Input: part model. Units: mm. Frame: model coordinates. Face numbers are marked on the shaded views. A direction names the side the tool comes from. Give positions to 0.01 mm unless a question says otherwise; leave off trailing zeros. Loops run counter-clockwise (first coordinate to the right, second up) from the corner with the lowest first, then second, coordinate; pieces in that order, holes last. Notation, with made-up numbers: M 46.25,59 L 51.25,59 A6 cw 51.25,67 Z; hole C 69.5,37.5 d2. An arc over 180 degrees is marked long. Answer as a JSON object with one key per item and string values. Group by question number.
1) Ray query, L1, parallel to X at y = 9, z = -96; L2, parallel to Z at x = -37.2, y = 10; L3, parallel to X at y = 14.25, z = -99. Return the intervals inside material, ascending.
2) First-contact query: P1, Ø6.5, axis at y = 10, z = -100, coming from the -X side; P2, Ø4, axis at x = 23, y = 8.5, coming from the -Z side; P3, Ø3, axis at y = 12, z = -98, coming from the +X side. Flat tips, straight axial feed; report the tip coordinate or a pass-through.
3) Access query for the marked faces 1 and 2. Directions: +Z, -Z, +X, -X, +Y, -Y. A direction counts if a zero-diameter tool reaches every point of the face in a straight line with its end or side. Return the directions, or none.
4) Section query B-B on x = 28.5. Return loops of the section in (y, z).
5) Section query A-A on z = -89. Return loops of the section in (x, y), plus the area to 3 significant figures.
6) Section query D-D on x = -7.5. Return loops of the section in (y, z), plus the area to 3 significant figures.
7) Section query C-C on z = -32. Return loops of the section in (x, y), plus the area to 3 significant figures.
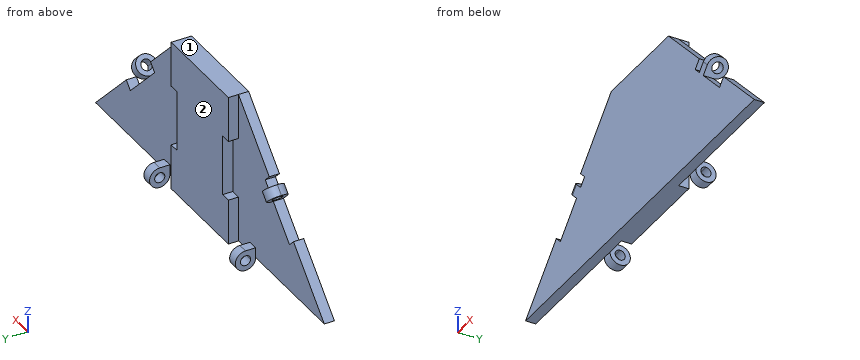
from build123d import *

# Parameters (mm, degrees)
BOSS_EXTRUDE1_DEPTH = 10
SKETCH2_W           = 5
SKETCH2_H           = 30
CUT_EXTRUDE1_DEPTH  = 5
CUT_EXTRUDE2_REACH  = 143.774
BOSS_EXTRUDE2_START = 5
BOSS_EXTRUDE2_DEPTH = 5
BOSS_EXTRUDE3_START = 10
BOSS_EXTRUDE3_DEPTH = 5


with BuildPart() as part:
    # Sketch1 → Boss-Extrude1 (new body)
    with BuildSketch(Plane(origin=(0, 0, 0), x_dir=(1, 0, 0), z_dir=(0, 1, 0))):
        Polygon((-25, 25), (-100, 100), (100, 100), (25, 25), align=None)
    extrude(amount=BOSS_EXTRUDE1_DEPTH)

    # Sketch2 → Cut-Extrude1 (cut)
    with BuildSketch(Plane(origin=(0, 10, 0), x_dir=(1, 0, 0), z_dir=(0, 1, 0))):
        Polygon((-25, 25), (-25, 47.5), (-25, 77.5), (-25, 100), (-100, 100), (-73.106601718, 73.106601718), (-69.571067812, 76.642135624), (-48.357864376, 55.428932188), (-51.893398282, 51.893398282), align=None)
        with Locations((-22.5, 62.5)):
            Rectangle(SKETCH2_W, SKETCH2_H)
    cut_extrude1 = extrude(amount=-CUT_EXTRUDE1_DEPTH, mode=Mode.SUBTRACT)

    # Sketch2_4 → Cut-Extrude2 (cut, up to next)
    with BuildSketch(Plane(origin=(0, 10, 0), x_dir=(1, 0, 0), z_dir=(0, 1, 0)), mode=Mode.PRIVATE) as cut_extrude2_sk1:
        Polygon((-73.106601718, 73.106601718), (-51.893398282, 51.893398282), (-48.357864376, 55.428932188), (-69.571067812, 76.642135624), align=None)
    cut_extrude2_tool1 = extrude(cut_extrude2_sk1.sketch, amount=-CUT_EXTRUDE2_REACH, mode=Mode.PRIVATE) & part.part
    cut_extrude2 = cut_extrude2_tool1.solids().sort_by_distance((-60.732233, 10, -64.267767))[0]
    add(cut_extrude2, mode=Mode.SUBTRACT)

    # Sketch3 → Boss-Extrude2 (add)
    with BuildSketch(Plane(origin=(-51.893398282, 0, -51.893398282), x_dir=(-0.7071067811865461, 0, 0.7071067811865489), z_dir=(-0.7071067811865489, 0, -0.7071067811865461)).offset(BOSS_EXTRUDE2_START)):
        with BuildLine():
            ThreePointArc((0, 0), (-3.535533906, 1.464466094), (-5, 5))
            Line((-5, 5), (-5, 0))
            Line((-5, 0), (0, 0))
        make_face()
        with BuildLine():
            ThreePointArc((0, 0), (3.535533906, 1.464466094), (5, 5))
            ThreePointArc((5, 5), (0, 10), (-5, 5))
            Line((-5, 5), (-2.634477445, 5))
            ThreePointArc((-2.634477445, 5), (0, 7.634477445), (2.634477445, 5))
            ThreePointArc((2.634477445, 5), (1.862856866, 3.137143134), (0, 2.365522555))
            Line((0, 2.365522555), (0, 0))
        make_face()
        with BuildLine():
            Line((-2.634477445, 5), (-5, 5))
            ThreePointArc((-5, 5), (-3.535533906, 1.464466094), (0, 0))
            Line((0, 0), (0, 2.365522555))
            ThreePointArc((0, 2.365522555), (-1.862856866, 3.137143134), (-2.634477445, 5))
        make_face()
    boss_extrude2 = extrude(amount=BOSS_EXTRUDE2_DEPTH)

    # Sketch4 → Boss-Extrude3 (add)
    with BuildSketch(Plane.ZY.offset(25).offset(BOSS_EXTRUDE3_START)):
        with BuildLine():
            Line((-97.5, 10), (-95, 10))
            ThreePointArc((-95, 10), (-103.535533906, 13.535533906), (-100, 5))
            Line((-100, 5), (-100, 7.5))
            ThreePointArc((-100, 7.5), (-101.767766953, 11.767766953), (-97.5, 10))
        make_face()
        with BuildLine():
            ThreePointArc((-100, 5), (-96.464466094, 6.464466094), (-95, 10))
            Line((-95, 10), (-97.5, 10))
            ThreePointArc((-97.5, 10), (-98.232233047, 8.232233047), (-100, 7.5))
            Line((-100, 7.5), (-100, 5))
        make_face()
        with BuildLine():
            Line((-95, 5), (-95, 10))
            ThreePointArc((-95, 10), (-96.464466094, 6.464466094), (-100, 5))
            Line((-100, 5), (-95, 5))
        make_face()
    boss_extrude3 = extrude(amount=BOSS_EXTRUDE3_DEPTH)

    # Mirror1: Cut-Extrude1, Cut-Extrude2, Boss-Extrude2, Boss-Extrude3 across plane
    add(cut_extrude1.mirror(Plane(origin=(0, 0, 0), x_dir=(0, 0, 1), z_dir=(1, 0, 0))), mode=Mode.SUBTRACT)
    add(cut_extrude2.mirror(Plane(origin=(0, 0, 0), x_dir=(0, 0, 1), z_dir=(1, 0, 0))), mode=Mode.SUBTRACT)
    add(boss_extrude2.mirror(Plane(origin=(0, 0, 0), x_dir=(0, 0, 1), z_dir=(1, 0, 0))))
    add(boss_extrude3.mirror(Plane(origin=(0, 0, 0), x_dir=(0, 0, 1), z_dir=(1, 0, 0))))


solid = part.part
Output:
{
 "1": {"L1": "x = -40 to -35, -25 to 25, 35 to 40", "L2": "z = -105 to -102.5, -97.5 to -95", "L3": "x = -40 to -35, 35 to 40"},
 "2": {"P1": "stops at x = -40", "P2": "stops at z = -100", "P3": "stops at x = 40"},
 "3": {"face 1": "+Z, +X, -X, +Y, -Y", "face 2": "+Z, -Z, +Y"},
 "4": {"outline": "M 0,-100 L 5,-100 L 5,-28.5 L 0,-28.5 Z"},
 "5": {"outline": "M -89,0 L 89,0 L 89,5 L 25,5 L 25,10 L -25,10 L -25,5 L -89,5 Z", "area": "1,140 mm^2"},
 "6": {"outline": "M 0,-100 L 10,-100 L 10,-25 L 0,-25 Z", "area": "750 mm^2"},
 "7": {"outline": "M -32,0 L 32,0 L 32,5 L 25,5 L 25,10 L -25,10 L -25,5 L -32,5 Z", "area": "570 mm^2"}
}
